from build123d import *

# Parameters (mm, degrees)
EXTRUDE_1_DEPTH     = 9
SKETCH_2_R          = 1.75
CUT_EXTRUDE_1_DEPTH = 5


with BuildPart() as part:
    # 草图1 → 凸台-拉伸1 (new body)
    with BuildSketch(Plane.XY):
        with BuildLine():
            Line((0, 0), (43, 0))
            Line((43, 0), (43, 16))
            ThreePointArc((43, 16), (32.200157728, 28.178005607), (17, 34))
            Line((17, 34), (0, 34))
            Line((0, 34), (0, 0))
        make_face()
    extrude(amount=EXTRUDE_1_DEPTH)

    # 草图2 → 切除-拉伸1 (cut)
    with BuildSketch(Plane.XZ):
        with Locations(Location((3.75, 3.75, 0), (0, 0, 270))):
            Circle(SKETCH_2_R)
        with Locations(Location((39.25, 3.75, 0), (0, 0, 90))):
            Circle(SKETCH_2_R)
    extrude(amount=-CUT_EXTRUDE_1_DEPTH, mode=Mode.SUBTRACT)


solid = part.part
Design review of the part built by this model. Coordinates are the model's own, in mm. A direction names the side the tool comes from. Round coordinates to 2 decimals unless told otherwise and drop trailing zeros. Write each loop counter-clockwise with the first axis right and the second up, starting at its lowest first coordinate (ties: lowest second). Pieces come first, ordered by that corner, then holes.
Item 1: For faces 1 (the cylindrical face through (40.96, 2.46, 3.37)), 2 (the flat face through (21, 17, 0)), list the 3-axis set-ups (+Z, -Z, +X, -X, +Y, -Y) from which the entire face can be reached by the end or side of a thin tool; tool diameter is ignored.
Item 2: Draft analysis for pull direction X (two halves, no side actions). For faces 3 (the flat face through (9, 34, 4)), 4 (the flat face through (39, 5, 4)), 5 (the cylindrical face through (2.69, 2.46, 5.14)), 6 (the cylindrical face through (32.389, 28.046, 4.437)), state which applies: released by +X, released by -X, zero draft, split by the parting line, or undercut.
Item 3: Consider section D-D on z = 1. Give the boundary of the cut face in (x, y), and give its area (3 significant figures).
Item 4: Consider section A-A on z = 3.75. Give the boundary of the cut face in (x, y), and give its area (3 significant figures).
Item 5: Consider section C-C on y = 20.5. Give the boundary of the cut face in (x, z), and give its area (3 significant figures).
Item 6: Consider section B-B on x = 3.75. Give the boundary of the cut face in (y, z), and give its area (4 significant figures).
Item 7: For pin 1 Ø2 at (x, z) = (3.75, 3.75) entering from -Y, flat-tipped, find the tip position at first contact; note if it passes through.
Item 8: Wall thickness on L1, parallel to X at y = 3.6, z = 3.75; L2, parallel to Z at x = 39.25, y = 3.2; L3, parallel to Z at x = 3, y = 1: over which ranges is each line inside the solid? List them lowest first.
Check values:
1. face 1: -Y
1. face 2: -Z, +X, -X, +Y, -Y
2. face 3: zero draft
2. face 4: undercut
2. face 5: undercut
2. face 6: released by +X
3. outline: (0, 0) - (43, 0) - (43, 16) arc R34.27 ccw to (17, 34) - (0, 34) - close
3. area: 1,310 mm2
4. outline: (0, 0) - (2, 0) - (2, 5) - (5.5, 5) - (5.5, 0) - (37.5, 0) - (37.5, 5) - (41, 5) - (41, 0) - (43, 0) - (43, 16) arc R34.27 ccw to (17, 34) - (0, 34) - close
4. area: 1,280 mm2
5. outline: (0, 0) - (40.16, 0) - (40.16, 9) - (0, 9) - close
5. area: 361 mm2
6. outline: (0, 0) - (34, 0) - (34, 9) - (0, 9) - (0, 5.5) - (5, 5.5) - (5, 2) - (0, 2) - close
6. area: 288.5 mm2
7. pin 1: stops at y = 5
8. L1: x = 0 to 2, 5.5 to 37.5, 41 to 43
8. L2: z = 0 to 2, 5.5 to 9
8. L3: z = 0 to 2.17, 5.33 to 9
